For this review, take the finished solid that the model builds, in its own axes (mm). A direction names the side the tool comes from. Round coordinates to 2 decimals unless told otherwise and drop trailing zeros. Loops run counter-clockwise (first coordinate to the right, second up) from the corner with the lowest first, then second, coordinate; pieces in that order, holes last.
1) Insertion check: pin 1 (4 mm diameter, centred on x = 1, y = 161, fed in from +Z). The pin has a flat end and moves straight along its axis. Give the tip position at first contact, or say it passes through.
2) Wall thickness on L1, parallel to Z at x = -14, y = 175; L2, parallel to X at y = 159.5, z = 10.5: over which ranges is each line inside the solid? List them lowest first.
3) Tool access review of faces 1 (the flat face through (1, 110, -18.114)), 2 (the flat face through (-19.014, 19.72, -0.394)): name each direction out of +Z, -Z, +X, -X, +Y, -Y from which nothing blocks a thin tool from reaching the whole face with its end or side.
4) Take a section at C-C (z = 3). State the section outline as (x, y) points.
5) Take a section at A-A (x = 1). State the section outline as (y, z) points.
6) Take a section at B-B (y = 67.5). State the section outline as (x, z) points, then the cut area to 3 significant figures.
```python
from build123d import *

# Parameters (mm, degrees)
BOSS_EXTRU_1_DEPTH      = 222
ENL_V_MAT_EXTRU_1_DEPTH = 590
ENL_V_MAT_EXTRU_2_DEPTH = 590


with BuildPart() as part:
    # Esquisse1 → Boss.-Extru.1 (new body)
    with BuildSketch(Plane(origin=(0, 0, 0), x_dir=(1, 0, 0), z_dir=(0, 1, 0))):
        Polygon((-20, 20.113636364), (20, 20.113636364), (20, 18.113636364), (-18, 18.113636364), (-18, -19.886363636), (-20, -19.886363636), align=None)
    extrude(amount=BOSS_EXTRU_1_DEPTH)

    # Esquisse2 → Enlèv. mat.-Extru.1 (cut)
    with BuildSketch(Plane(origin=(0, 0, -20.113636364), x_dir=(-1, 0, 0), z_dir=(0, 0, -1))):
        Polygon((20, 0), (-20, 40), (-20, 0), align=None)
    extrude(amount=-ENL_V_MAT_EXTRU_1_DEPTH, mode=Mode.SUBTRACT)

    # Esquisse3 → Enlèv. mat.-Extru.2 (cut)
    with BuildSketch(Plane.ZY.offset(20)):
        Polygon((-20.113636364, 0), (19.886363636, 40), (19.886363636, 0), align=None)
    extrude(amount=-ENL_V_MAT_EXTRU_2_DEPTH, mode=Mode.SUBTRACT)


solid = part.part
```
Response:
1. pin 1: stops at z = -18.11
2. L1: z = -20.11 to -18.11
2. L2: x = -20 to -18
3. face 1: +Z, +X, +Y, -Y
3. face 2: +Z, +X, -X, -Y
4. outline: (-20, 23.11) - (-18, 23.11) - (-18, 222) - (-20, 222) - close
5. outline: (21, -20.11) - (222, -20.11) - (222, -18.11) - (21, -18.11) - close
6. outline: (-20, -20.11) - (20, -20.11) - (20, -18.11) - (-18, -18.11) - (-18, 19.89) - (-20, 19.89) - close
6. area: 156 mm2
